from build123d import *

# Parameters (mm, degrees)
BOSS_EXTRUDE1_DEPTH              = 50.8
SKETCH2_R                        = 7.9375
CUT_EXTRUDE1_DEPTH               = 12.7
F_10_CLEARANCE_HOLE1_D           = 5.1054
F_10_CLEARANCE_HOLE1_ON_FACE_2_D = 5.1054
CUT_EXTRUDE4_DEPTH               = 57


with BuildPart() as part:
    # Sketch1 → Boss-Extrude1 (new body)
    with BuildSketch(Plane.XY):
        with BuildLine():
            Line((23.736970149, 16.573322883), (45.005970149, 16.573322883))
            Line((45.005970149, 16.573322883), (45.005970149, -2.476677117))
            Line((45.005970149, -2.476677117), (-10.994029851, -2.476677117))
            Line((-10.994029851, -2.476677117), (-10.994029851, 16.573322883))
            Line((-10.994029851, 16.573322883), (10.274970149, 16.573322883))
            ThreePointArc((10.274970149, 16.573322883), (17.005970149, 9.842322883), (23.736970149, 16.573322883))
        make_face()
    extrude(amount=BOSS_EXTRUDE1_DEPTH)

    # Sketch2 → Cut-Extrude1 (cut, symmetric)
    with BuildSketch(Plane.XY.offset(25.4)):
        with Locations((17.005970149, 16.573322883)):
            Circle(SKETCH2_R)
    extrude(amount=CUT_EXTRUDE1_DEPTH, both=True, mode=Mode.SUBTRACT)

    # #10 Clearance Hole1 (through all)
    with Locations(Plane(origin=(-10.994029851, 3.873322883, 41.402), x_dir=(0, 0, -1), z_dir=(-1, 0, 0))):
        with Locations((0, 0), (32.004, 0)):
            Hole(F_10_CLEARANCE_HOLE1_D / 2)

    # #10 Clearance Hole1 on face 2 (through all)
    with Locations(Plane(origin=(-1.596029851, 11.493322883, 50.8), x_dir=(1, 0, 0), z_dir=(0, 0, 1))):
        with Locations((0, 0), (37.204, 0)):
            Hole(F_10_CLEARANCE_HOLE1_ON_FACE_2_D / 2)

    # Sketch9 → Cut-Extrude4 (cut, through all)
    with BuildSketch(Plane(origin=(45.005970149, 0, 0), x_dir=(0, 0, -1), z_dir=(1, 0, 0))):
        with BuildLine():
            Line((-32.512, -2.476677117), (-18.288, -2.476677117))
            ThreePointArc((-18.288, -2.476677117), (-25.4, 4.635322883), (-32.512, -2.476677117))
        make_face()
    extrude(amount=-CUT_EXTRUDE4_DEPTH, mode=Mode.SUBTRACT)


solid = part.part
CAD build for the part. Positions are in the model's coordinates, mm. A direction names the side the tool comes from. Coordinates: 2 decimals unless noted, no trailing zeros. Order: outer loops, then holes, each group sorted by start corner. A loop starts at its lowest first (then second) coordinate and runs counter-clockwise, first axis right, second up. Notation, with made-up numbers: (-12.75, 56.25) -> (28.25, 56.25) arc R11 ccw to (28.25, 75.25) -> close; hole circle Ø11 at (50, -28.75). An arc over 180 degrees is marked (long way). Answer in a Markdown table with one row per item.
1) Which spindle directions (+Z, -Z, +X, -X, +Y, -Y) get a long thin tool onto all of the face, cutting with end or side? Do faces 5 (the face through (16.858, 9.844, 6.261)), 6 (the face through (16.97, 9.68, 12.7)). Say none if no direction does.
Check values:
| item | result |
|---|---|
| face 5 | +Z, -Z, +Y |
| face 6 | +Y |
2) Flat gauge pins, fed straight in: P1, Ø3, axis at x = 14.5, z = 6.5, coming from the +Y side; P2, Ø6, axis at x = 38.5, z = 28, coming from the -Y side. Where does each tip first touch, or does it go through?
Check values:
| item | result |
|---|---|
| P1 | y = 11.16 |
| P2 | y = 1.91 |
3) Mould opens along Z. For faces 1 (the face through (16.831, 8.638, 25.578)), 2 (the face through (17.4, 3.76, 38.85)), 3 (the face through (34, 16.573, 25)), 4 (the face through (17, 7, 0)) say: pulls with the +Z half, pulls with the -Z half, needs draft (parallel to the pull), parting line crosses it, or undercut.
Check values:
| item | result |
|---|---|
| face 1 | undercut |
| face 2 | undercut |
| face 3 | needs draft |
| face 4 | pulls with the -Z half |
4) Band-saw the part on A-A (z = 11). List the corners of the cut face in (x, y).
Check values:
| item | result |
|---|---|
| outline | (-10.99, -2.48) -> (45.01, -2.48) -> (45.01, 1.89) -> (-10.99, 1.89) -> close; (-10.99, 5.86) -> (45.01, 5.86) -> (45.01, 16.57) -> (23.74, 16.57) arc R6.73 cw to (10.27, 16.57) -> (-10.99, 16.57) -> close; hole circle Ø5.11 at (-1.6, 11.49); hole circle Ø5.11 at (35.61, 11.49) |
5) Band-saw the part on B-B (x = 35). List the corners of the cut face in (y, z).
Check values:
| item | result |
|---|---|
| outline | (-2.48, 0) -> (9.01, 0) -> (9.01, 50.8) -> (-2.48, 50.8) -> (-2.48, 32.51) arc R7.11 cw to (-2.48, 18.29) -> close; (13.97, 0) -> (16.57, 0) -> (16.57, 50.8) -> (13.97, 50.8) -> close; hole circle Ø5.11 at (3.87, 9.4); hole circle Ø5.11 at (3.87, 41.4) |
6) Drill centre lines: line 1 (X direction, y = 12.25, z = 40); line 2 (Y direction, x = 10, z = 9.5); line 3 (X direction, y = 13.25, z = 20). Where is each one in solid material? Low to high.
Check values:
| item | result |
|---|---|
| line 1 | -10.99 to -4.03, 0.84 to 11.85, 22.16 to 33.17, 38.05 to 45.01 |
| line 2 | -2.48 to 1.32, 6.42 to 16.57 |
| line 3 | -10.99 to -3.45, 0.26 to 9.8, 24.21 to 33.76, 37.46 to 45.01 |
7) Band-saw the part on D-D (z = 34.5). List the corners of the cut face in (x, y) (1 decimal).
Check values:
| item | result |
|---|---|
| outline | (-11, -2.5) -> (45, -2.5) -> (45, 16.6) -> (24.9, 16.6) arc R7.9 cw to (9.1, 16.6) -> (-11, 16.6) -> close; hole circle Ø5.1 at (-1.6, 11.5); hole circle Ø5.1 at (35.6, 11.5) |
8) Band-saw the part on C-C (x = -5). List the corners of the cut face in (y, z).
Check values:
| item | result |
|---|---|
| outline | (-2.48, 0) -> (16.57, 0) -> (16.57, 50.8) -> (-2.48, 50.8) -> (-2.48, 32.51) arc R7.11 cw to (-2.48, 18.29) -> close; hole circle Ø5.11 at (3.87, 9.4); hole circle Ø5.11 at (3.87, 41.4) |
